from build123d import *

# Parameters (mm, degrees)
F2_R     = 9
F3_DEPTH = 37
F4_SIZE  = 0.8
F5_R     = 1.6


with BuildPart() as f1:
    # F0 (on Front) → F1 (revolve)
    with BuildSketch(Plane.XZ):
        Polygon((-17, -16.36958538), (-27, -16.36958538), (-27, -30.36958538), (10, -30.36958538), (10, -16.36958538), (0, -16.36958538), (0, -27.36958538), (-17, -27.36958538), align=None)
    revolve(axis=Axis((-22, 0, -16.36958538), (1, 0, 0)))

    # F2 (on face) → F3 (cut)
    with BuildSketch(Plane.YZ.offset(10)):
        with Locations((0, -16.36958538)):
            Circle(F2_R)
    extrude(amount=-F3_DEPTH, mode=Mode.SUBTRACT)

    # F4
    f4_edges = [f1.edges().sort_by_distance(p)[0] for p in [
        (10, 0, -2.369585),
        (-27, 0, -2.369585),
    ]]
    chamfer(f4_edges, length=F4_SIZE)

    # F5
    f5_edges = [f1.edges().sort_by_distance(p)[0] for p in [
        (-17, 0, -5.369585),
        (0, 0, -5.369585),
    ]]
    fillet(f5_edges, radius=F5_R)


solid = f1.part
CAD build for the part. Positions are in the model's coordinates, mm. A direction names the side the tool comes from. Give positions to 0.01 mm unless a question says otherwise; leave off trailing zeros. Loops run counter-clockwise (first coordinate to the right, second up) from the corner with the lowest first, then second, coordinate; pieces in that order, holes last. Notation, with made-up numbers: M 5,59 L 27,59 A12 cw 27,81 Z; hole C 71,70 d2. An arc over 180 degrees is marked long. Write each question's results on one line, items separated by ' | '.
Q1. Probe probe 1 along Z at (x, y) = (-2.5, 0.25); probe 2 along Y at (x, z) = (-21.5, -22); probe 3 along Y at (x, z) = (-18, -9.75). List the from-to ranges inside material, lowest first.
Geometry check:
probe 1: z = -30.37 to -27.37, -5.37 to -2.37 | probe 2: y = -12.82 to -7.02, 7.02 to 12.82 | probe 3: y = -12.34 to -6.1, 6.1 to 12.34
Q2. Mould opens along Z. For faces 3 (the face through (-27, -9, -14)), 4 (the face through (5.07, -1.172, -7.446)), 5 (the face through (-8.25, 4.21, -29.72)) say: pulls with the +Z half, pulls with the -Z half, needs draft (parallel to the pull), parting line crosses it, or undercut.
Geometry check:
face 3: needs draft | face 4: undercut | face 5: parting line crosses it
Q3. Flat gauge pins, fed straight in: P1, Ø12, axis at x = -4.5, z = -5, coming from the -Y side; P2, Ø3, axis at x = 4.5, y = 10.5, coming from the +Z side; P3, Ø1, axis at x = -1, z = -19, coming from the +Y side. Where does each tip first touch, or does it go through?
Geometry check:
P1: stops at y = -12.93 | P2: stops at z = -5.65 | P3: stops at y = 13.84
Q4. Which spindle directions (+Z, -Z, +X, -X, +Y, -Y) get a long thin tool onto all of the face, cutting with end or side? Do faces 1 (the face through (-17, -8, -21)), 2 (the face through (-21.93, -1.172, -7.446)). Say none if no direction does.
Geometry check:
face 1: none | face 2: +X, -X
Q5. Band-saw the part on B-B on x = -19. Write the cut outline in (y, z).
Geometry check:
outline: C 0,-16.37 d28; hole C 0,-16.37 d18
Q6. Band-saw the part on A-A on y = 0. Write the cut outline in (x, z).
Geometry check:
outline: M -27,-29.57 L -26.2,-30.37 L 9.2,-30.37 L 10,-29.57 L 10,-25.37 L 0,-25.37 L 0,-25.77 A1.6 cw -1.6,-27.37 L -15.4,-27.37 A1.6 cw -17,-25.77 L -17,-25.37 L -27,-25.37 Z; M -27,-7.37 L -17,-7.37 L -17,-6.97 A1.6 cw -15.4,-5.37 L -1.6,-5.37 A1.6 cw 0,-6.97 L 0,-7.37 L 10,-7.37 L 10,-3.17 L 9.2,-2.37 L -26.2,-2.37 L -27,-3.17 Z
